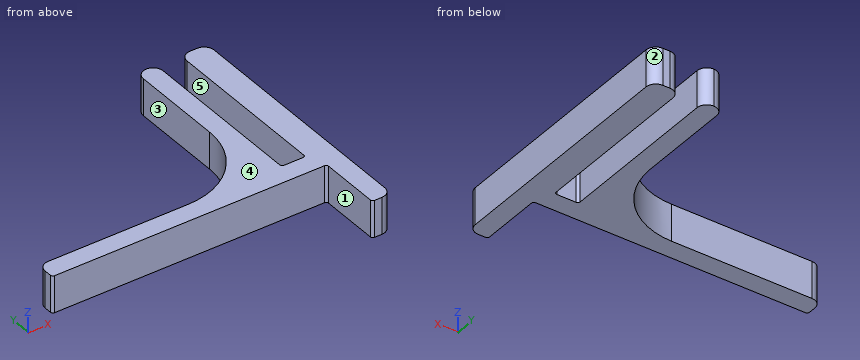
```python
from build123d import *

# Parameters (mm, degrees)
F1_DEPTH = 7.5
F2_R     = 1.99999
F3_R     = 15
F4_R     = 0.5


# Not quite as in the source:
# - a fillet or chamfer is up to 0.001 mm smaller than in the source, because OpenCascade refuses the exact size


with BuildPart() as f1:
    # F0 (on Top) → F1 (new body)
    with BuildSketch(Plane.XY):
        Polygon((45.6, 4), (0, 4), (0, 0), (56, 0), (56, -13), (60, -13), (60, 40), (54.5, 40), (54.5, 4), (49.6, 4), (49.6, 40), (45.6, 40), align=None)
    extrude(amount=F1_DEPTH)

    # F2 (radius 2 in the source; OpenCascade refuses exactly that, so slightly less here)
    f2_edges = [f1.edges().sort_by_distance(p)[0] for p in [
        (60, -13, 3.75),
        (60, 40, 3.75),
        (54.5, 40, 3.75),
        (49.6, 40, 3.75),
        (45.6, 40, 3.75),
        (0, 4, 3.75),
    ]]
    fillet(f2_edges, radius=F2_R)

    # F3
    f3_edges = [f1.edges().sort_by_distance(p)[0] for p in [
        (45.6, 4, 3.75),
    ]]
    fillet(f3_edges, radius=F3_R)

    # F4
    f4_edges = [f1.edges().sort_by_distance(p)[0] for p in [
        (49.6, 4, 3.75),
        (54.5, 4, 3.75),
        (0, 0, 3.75),
        (56, -13, 3.75),
        (56, 0, 3.75),
    ]]
    fillet(f4_edges, radius=F4_R)


solid = f1.part
```
Read the model definition and answer for the solid it produces. Units are mm, in the model's axes. Face numbers are marked on the shaded views. A direction names the side the tool comes from. Round coordinates to 2 decimals unless told otherwise and drop trailing zeros. Write each loop counter-clockwise with the first axis right and the second up, starting at its lowest first coordinate (ties: lowest second). Pieces come first, ordered by that corner, then holes. Notation, with made-up numbers: (56, 63) - (62, 63) arc R30 ccw to (62, 95) - close; hole circle Ø3 at (-36, -4.5). An arc over 180 degrees is marked (long way). One line per item, written item: value.
Q1. Find section C-C (x = 10). Determine the outline of the cut face in (y, z), and give its area (3 significant figures).
The answers:
outline: (0, 0) - (4, 0) - (4, 7.5) - (0, 7.5) - close
area: 30.0 mm2
Q2. Which of the six approach directions +Z, -Z, +X, -X, +Y, -Y give full straight-line access (tool end or side, diameter ignored) to the marked faces 1, 2, 3, 4 and 5?
The answers:
face 1: +Z, -Z, -X, -Y
face 2: +Z, -Z, +X, +Y
face 3: +Z, -Z, -X, +Y
face 4: +Z, +X, -X, +Y, -Y
face 5: +Z, -Z, +Y
Q3. Straight lines are drawn through the part: line 1 (X direction, y = 27.5, z = 2); line 2 (Y direction, x = 15, z = 2.75); line 3 (X direction, y = 9, z = 4.5). For each, find the intervals that lie inside material, in ascending order. Write a range as from..to.
The answers:
line 1: x = 45.6..49.6, 54.5..60
line 2: y = 0..4
line 3: x = 41.78..49.6, 54.5..60
Q4. Find section A-A (y = 32.5). Determine the outline of the cut face in (x, z), and give its area (4 significant figures).
The answers:
outline: (45.6, 0) - (49.6, 0) - (49.6, 7.5) - (45.6, 7.5) - close; (54.5, 0) - (60, 0) - (60, 7.5) - (54.5, 7.5) - close
area: 71.25 mm2
Q5. Each of these flat-tipped pins is pushed along its axis until it touches: P1, Ø1, axis at y = -2.5, z = 6.5, coming from the -X side; P2, Ø2, axis at x = 33.5, z = 4, coming from the -Y side; P3, Ø4, axis at x = 20.5, z = 4.5, coming from the +Y side. Where does it stop, or does it pass through?
The answers:
P1: stops at x = 56
P2: stops at y = 0
P3: stops at y = 4
Q6. Find section D-D (y = -9). Determine the outline of the cut face in (x, z), and give its area (3 significant figures).
The answers:
outline: (56, 0) - (60, 0) - (60, 7.5) - (56, 7.5) - close
area: 30.0 mm2
